from build123d import *

# Parameters (mm, degrees)
SKETCH1_W           = 8.85
SKETCH1_H           = 23.1
BOSS_EXTRUDE1_DEPTH = 2
BOSS_EXTRUDE2_DEPTH = 3.59
BOSS_EXTRUDE3_DEPTH = 4


with BuildPart() as part:
    # Sketch1 → Boss-Extrude1 (new body)
    with BuildSketch(Plane.XY):
        Polygon((0, 81.3), (0, 0), (40, 0), (40, 13.5), (25.35, 13.5), (25.35, 67.8), (64.65, 67.8), (64.65, 13.5), (50, 13.5), (50, 0), (90, 0), (90, 81.3), align=None)
        with Locations((82.575, 14.55)):
            Rectangle(SKETCH1_W, SKETCH1_H, mode=Mode.SUBTRACT)
        with Locations((82.575, 40.65)):
            Rectangle(SKETCH1_W, SKETCH1_H, mode=Mode.SUBTRACT)
        with Locations((82.575, 66.75)):
            Rectangle(SKETCH1_W, SKETCH1_H, mode=Mode.SUBTRACT)
        with Locations((7.425, 66.75)):
            Rectangle(SKETCH1_W, SKETCH1_H, mode=Mode.SUBTRACT)
        with Locations((7.425, 40.65)):
            Rectangle(SKETCH1_W, SKETCH1_H, mode=Mode.SUBTRACT)
        with Locations((7.425, 14.55)):
            Rectangle(SKETCH1_W, SKETCH1_H, mode=Mode.SUBTRACT)
    extrude(amount=BOSS_EXTRUDE1_DEPTH)

    # Sketch1<3> → Boss-Extrude2 (add)
    with BuildSketch(Plane.XY):
        Polygon((14.85, 3), (40, 3), (40, 10.5), (22.35, 10.5), (22.35, 70.8), (67.65, 70.8), (67.65, 10.5), (50, 10.5), (50, 3), (75.15, 3), (75.15, 78.3), (14.85, 78.3), align=None)
    extrude(amount=BOSS_EXTRUDE2_DEPTH)

    # Sketch1<4> → Boss-Extrude3 (add)
    with BuildSketch(Plane.XY):
        Polygon((11.85, 3), (11.85, 0), (40, 0), (40, 3), (14.85, 3), (14.85, 78.3), (75.15, 78.3), (75.15, 3), (50, 3), (50, 0), (78.15, 0), (78.15, 3), (78.15, 26.1), (78.15, 29.1), (78.15, 52.2), (78.15, 55.2), (78.15, 78.3), (78.15, 81.3), (11.85, 81.3), (11.85, 78.3), (11.85, 55.2), (11.85, 52.2), (11.85, 29.1), (11.85, 26.1), align=None)
    extrude(amount=BOSS_EXTRUDE3_DEPTH)


solid = part.part
Can you work these out from the model? Positions are in its coordinate system, mm. A direction names the side the tool comes from. Give positions to 0.01 mm unless a question says otherwise; leave off trailing zeros. Write each loop counter-clockwise with the first axis right and the second up, starting at its lowest first coordinate (ties: lowest second). Pieces come first, ordered by that corner, then holes. Notation, with made-up numbers: M 54.25,89 L 111.25,89 A26 cw 111.25,128 Z; hole C 4,57 d6. An arc over 180 degrees is marked long. Answer in a Markdown table with one row per item. Add a question column.
Item 1: Imagine slicing it at D-D, the plane z = 0.7. State how many separate pieces and enclosed holes the cut face has, plus the area to 3 significant figures.
Item 2: Imagine slicing it at B-B, the plane x = 82.5. Write out the boundary of the cut face in (y, z), plus the area to 3 significant figures.
Item 3: On a 3-axis mill with a long thin cutter (end or side, diameter ignored), from which of +Z, -Z, +X, -X, +Y, -Y can I reach the whole of each face in a straight line? I mean faces 1 (the flat face through (7, 78.3, 1)), 2 (the flat face through (25, 43, 2)), 3 (the flat face through (88, 41, 2)), 4 (the flat face through (50, 7, 2)). Say none if no direction works.
Item 4: For pin 1 Ø18 at (x, y) = (58.5, 26) entering from +Z, with a flat end and sliding along its axis, tell me the tip position at first contact or that it passes through.
Item 5: Please list where these lines run through material, in increasing order: L1, parallel to X at y = 48, z = 1; L2, parallel to Y at x = 83, z = 0.55; L3, parallel to X at y = 4.5, z = 0.45.
Item 6: Imagine slicing it at C-C, the plane y = 16.5. Write out the boundary of the cut face in (x, z), plus the area to 3 significant figures.
Item 7: Imagine slicing it at A-A, the plane x = 57.5. Write out the boundary of the cut face in (y, z).
Evaluation:
| question | item | result |
|---|---|---|
| 1 | separate pieces | 1 |
| 1 | enclosed holes | 6 |
| 1 | area | 3,820 mm² |
| 2 | outline | M 0,0 L 3,0 L 3,2 L 0,2 Z; M 26.1,0 L 29.1,0 L 29.1,2 L 26.1,2 Z; M 52.2,0 L 55.2,0 L 55.2,2 L 52.2,2 Z; M 78.3,0 L 81.3,0 L 81.3,2 L 78.3,2 Z |
| 2 | area | 24.0 mm² |
| 3 | face 1 | +Z, -Z |
| 3 | face 2 | +Z |
| 3 | face 3 | +Z, +X, +Y, -Y |
| 3 | face 4 | +Z, -Z, -Y |
| 4 | pin 1 | stops at z = 2 |
| 5 | L1 | x = 0 to 3, 11.85 to 25.35, 64.65 to 78.15, 87 to 90 |
| 5 | L2 | y = 0 to 3, 26.1 to 29.1, 52.2 to 55.2, 78.3 to 81.3 |
| 5 | L3 | x = 0 to 3, 11.85 to 40, 50 to 78.15, 87 to 90 |
| 6 | outline | M 0,0 L 3,0 L 3,2 L 0,2 Z; M 11.85,0 L 25.35,0 L 25.35,2 L 22.35,2 L 22.35,3.59 L 14.85,3.59 L 14.85,4 L 11.85,4 Z; M 64.65,0 L 78.15,0 L 78.15,4 L 75.15,4 L 75.15,3.59 L 67.65,3.59 L 67.65,2 L 64.65,2 Z; M 87,0 L 90,0 L 90,2 L 87,2 Z |
| 6 | area | 102 mm² |
| 7 | outline | M 0,0 L 13.5,0 L 13.5,2 L 10.5,2 L 10.5,3.59 L 3,3.59 L 3,4 L 0,4 Z; M 67.8,0 L 81.3,0 L 81.3,4 L 78.3,4 L 78.3,3.59 L 70.8,3.59 L 70.8,2 L 67.8,2 Z |
